Verification items for this drawing (mm, ordinates from the low corner). Round coordinates to 2 decimals unless told otherwise and drop trailing zeros. Loops run counter-clockwise (first coordinate to the right, second up) from the corner with the lowest first, then second, coordinate; pieces in that order, holes last. Notation, with made-up numbers: (5.5, 84.5) - (14.5, 84.5) arc R23 ccw to (14.5, 103.5) - close; hole circle Ø10 at (81.25, 61). An arc over 180 degrees is marked (long way). Answer in a Markdown table with one row per item. Add a question column.
(1) Cross-section at A-A on x = 5. Enter the section's corners in (y, z), then the cut area to 3 significant figures.
(2) Mould release check, pull along X, two halves, no side actions. Record for the marked faces 1, 2 and 3: +X half, -X half, draft (parallel to the pull), parting line (faces both ways), or undercut.
(3) Cross-section at C-C on z = 6.75. Enter the section's corners in (x, y).
(4) Thickness scan on line 1 along X through (y, z) = (5, 9.25). Record the ranges inside material, lowest first.
(5) Gauge pin test, flat end, axial feed: pin 1 (2.5 mm diameter, centred on x = 5, y = 5, fed in from +Z). Record the tip position at first contact, or that the pin passes through.
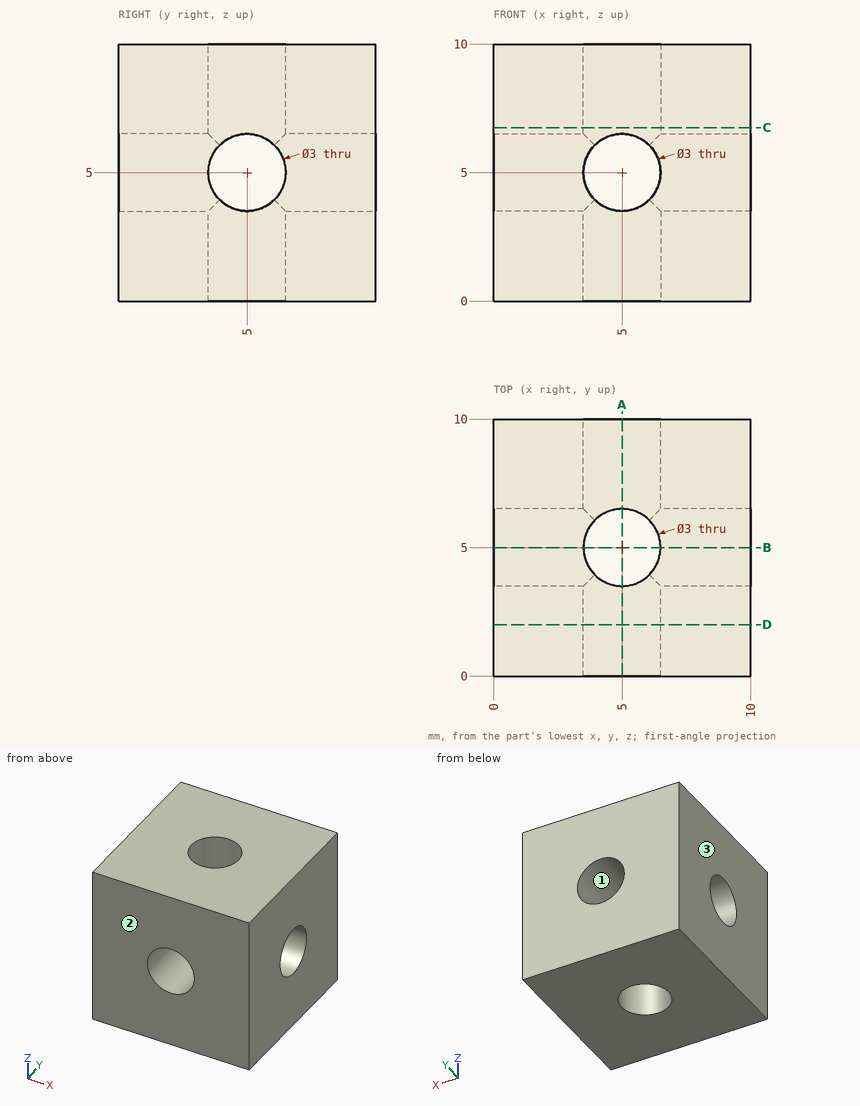
Answers:
| question | item | result |
|---|---|---|
| 1 | outline | (0, 0) - (3.5, 0) - (3.5, 3.5) - (0, 3.5) - close; (0, 6.5) - (3.5, 6.5) - (3.5, 10) - (0, 10) - close; (6.5, 0) - (10, 0) - (10, 3.5) - (6.5, 3.5) - close; (6.5, 6.5) - (10, 6.5) - (10, 10) - (6.5, 10) - close |
| 1 | area | 49.0 mm^2 |
| 2 | face 1 | undercut |
| 2 | face 2 | draft |
| 2 | face 3 | -X half |
| 3 | outline | (0, 0) - (10, 0) - (10, 10) - (0, 10) - close; hole circle Ø3 at (5, 5) |
| 4 | line 1 | x = 0 to 3.5, 6.5 to 10 |
| 5 | pin 1 | passes through |
